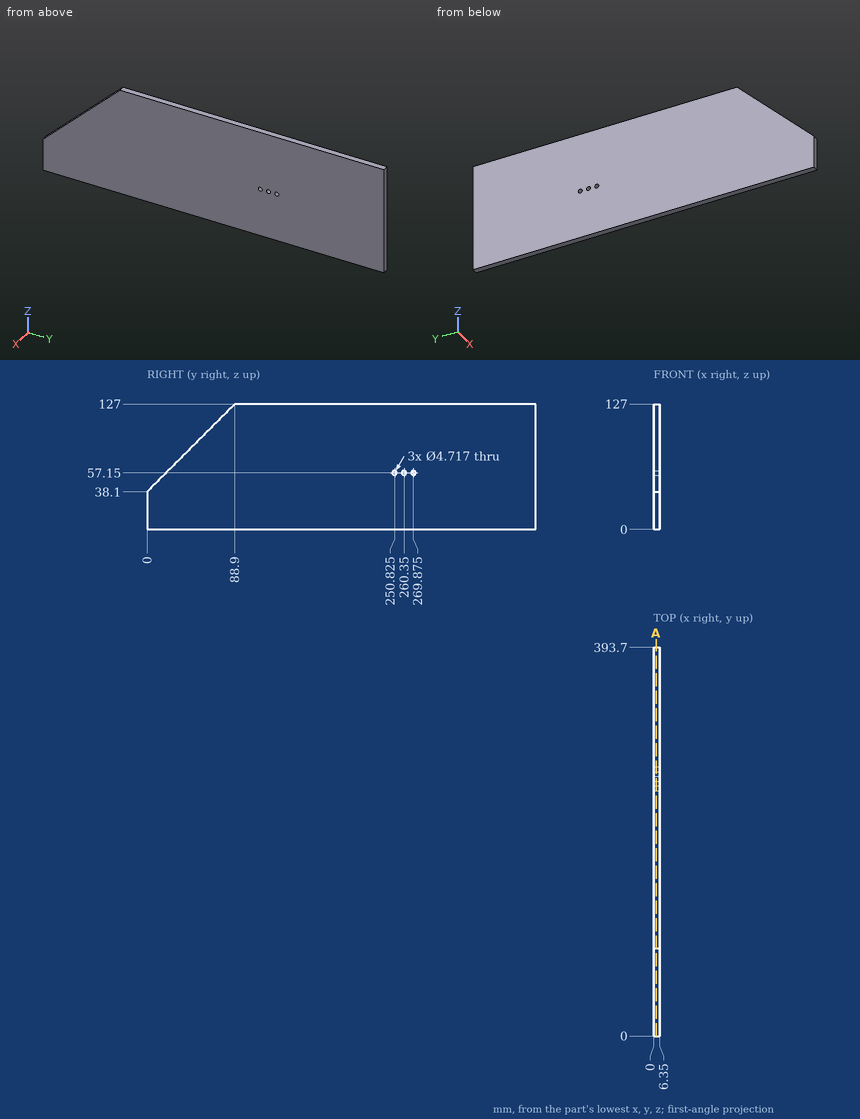
Could you check a few things on this drawing? It's one solid part, dimensions in mm from its lowest x, y, z. Give positions to 0.01 mm unless a question says otherwise; leave off trailing zeros. Return JSON: item names as keys, results as strings. Group by question number.
Q1. Will this pin go through, and if not, where does the flat tip stop? pin 1 Ø4 at (y, z) = (269.875, 57.15) entering from -X.
Q2. Suppose I cut it at A-A, the plane x = 2.5. State how many separate pieces and enclosed holes the cut face has, and give its area (3 significant figures).
Q3. Please list where these lines run through material, in increasing order: line 1 along Z through (x, y) = (4.25, 260.35); line 2 along Z through (x, y) = (0.5, 46); line 3 along Y through (x, z) = (5, 80). Write a range as [from, to].
Resolved:
{
 "1": {"pin 1": "passes through"},
 "2": {"separate pieces": "1", "enclosed holes": "3", "area": "46,000 mm2"},
 "3": {"line 1": "z = [0, 54.79], [59.51, 127]", "line 2": "z = [0, 84.1]", "line 3": "y = [41.9, 393.7]"}
}
